```python
from build123d import *

# Parameters (mm, degrees)
SKETCH_1_W                    = 380
SKETCH_1_H                    = 380
EXTRUDE_1_DEPTH               = 14
CHAMFER_1_SIZE                = 2
HOLE_WIZARD_M8_1_D            = 6.8
HOLE_WIZARD_M10_1_D           = 11
HOLE_WIZARD_M10_1_CBORE_D     = 22
HOLE_WIZARD_M10_1_CBORE_DEPTH = 10.5
SKETCH_6_R                    = 8
CUT_EXTRUDE_1_DEPTH           = 15


with BuildPart() as part:
    # 草图1 → 凸台-拉伸1 (new body)
    with BuildSketch(Plane(origin=(0, 0, 0), x_dir=(1, 0, 0), z_dir=(0, 1, 0))):
        Rectangle(SKETCH_1_W, SKETCH_1_H)
    extrude(amount=EXTRUDE_1_DEPTH)

    # 倒角1
    chamfer_1_edges = [part.edges().sort_by_distance(p)[0] for p in [
        (-190, 7, -190),
        (190, 7, -190),
        (190, 7, 190),
        (-190, 7, 190),
    ]]
    chamfer(chamfer_1_edges, length=CHAMFER_1_SIZE)

    # M8 螺纹孔的螺纹孔钻头1 (through all)
    with Locations(Plane(origin=(0, 14, 0), x_dir=(1, 0, 0), z_dir=(0, 1, 0))):
        with Locations((60, 40), (60, 0), (60, -40)):
            hole_wizard_m8_1 = Hole(HOLE_WIZARD_M8_1_D / 2)

    # 镜向1: M8 螺纹孔的螺纹孔钻头1 across plane
    add(hole_wizard_m8_1.mirror(Plane(origin=(0, 0, 0), x_dir=(0, 0, 1), z_dir=(1, 0, 0))), mode=Mode.SUBTRACT)

    # M10 六角头螺栓的柱形沉头孔1 (through all)
    with Locations(Plane(origin=(0, 0, 0), x_dir=(-1, 0, 0), z_dir=(0, -1, 0))):
        with Locations((33.5, 53.5), (-33.5, -13.5), (33.5, -53.5), (-33.5, 53.5), (-33.5, -53.5), (33.5, 13.5)):
            CounterBoreHole(HOLE_WIZARD_M10_1_D / 2, HOLE_WIZARD_M10_1_CBORE_D / 2, HOLE_WIZARD_M10_1_CBORE_DEPTH)

    # 草图6 → 切除-拉伸1 (cut, through all)
    with BuildSketch(Plane(origin=(0, 14, 0), x_dir=(1, 0, 0), z_dir=(0, 1, 0))):
        with Locations((-162, 162)):
            Circle(SKETCH_6_R)
        with Locations((162, 162)):
            Circle(SKETCH_6_R)
        with Locations((-162, -162)):
            Circle(SKETCH_6_R)
        with Locations((162, -162)):
            Circle(SKETCH_6_R)
    extrude(amount=-CUT_EXTRUDE_1_DEPTH, mode=Mode.SUBTRACT)


solid = part.part
```
Read the model definition and answer for the solid it produces. Units are mm, in the model's axes. A direction names the side the tool comes from. Give positions to 0.01 mm unless a question says otherwise; leave off trailing zeros. Write each loop counter-clockwise with the first axis right and the second up, starting at its lowest first coordinate (ties: lowest second). Pieces come first, ordered by that corner, then holes. Notation, with made-up numbers: M 48,-19.5 L 74,-19.5 A21 cw 74,12.5 Z; hole C 65.5,-20.75 d7. An arc over 180 degrees is marked long. Put each result on its own line as item: value. Start each with the question number.
1. The part is cut by section C-C, the plane y = 8. Give the number of separate pieces and of enclosed holes in the cut face, and give its area (3 significant figures).
2. The part is cut by section B-B, the plane x = 162. Give the vertices of the cut face in (y, z), and give its area (3 significant figures).
3. Each of these flat-tipped pins is pushed along its axis until it touches: pin 1 Ø13 at (x, z) = (-162, 162) entering from -Y; pin 2 Ø24 at (x, z) = (32.5, 12.5) entering from -Y; pin 3 Ø20 at (x, z) = (-33.5, -53.5) entering from -Y. Where does it stop, or does it pass through?
4. The part is cut by section D-D, the plane x = -33.5. Give the vertices of the cut face in (y, z).
5. Which of the six approach directions +Z, -Z, +X, -X, +Y, -Y give full straight-line access (tool end or side, diameter ignored) to faces 1 (the cylindrical face through (-38.995, 12.274, -53.742)), 2 (the flat face through (-28, 10.5, -51))?
6. Consider line 1 along Z through (x, y) = (-33.5, 4.5); line 2 along Z through (x, y) = (-60, 9.75); line 3 along X through (y, z) = (13.35, -53.5). Determine where each line is inside the solid, lowest interval first.
7. The part is cut by section A-A, the plane z = 162. Give the vertices of the cut face in (x, y).
Final values:
1. separate pieces: 1
1. enclosed holes: 16
1. area: 141,000 mm²
2. outline: M 0,-190 L 14,-190 L 14,-170 L 0,-170 Z; M 0,-154 L 14,-154 L 14,154 L 0,154 Z; M 0,170 L 14,170 L 14,190 L 0,190 Z
2. area: 4,870 mm²
3. pin 1: passes through
3. pin 2: stops at y = 0
3. pin 3: stops at y = 10.5
4. outline: M 0,-190 L 14,-190 L 14,-59 L 10.5,-59 L 10.5,-64.5 L 0,-64.5 Z; M 0,-42.5 L 10.5,-42.5 L 10.5,-48 L 14,-48 L 14,-19 L 10.5,-19 L 10.5,-24.5 L 0,-24.5 Z; M 0,-2.5 L 10.5,-2.5 L 10.5,-8 L 14,-8 L 14,48 L 10.5,48 L 10.5,42.5 L 0,42.5 Z; M 0,64.5 L 10.5,64.5 L 10.5,59 L 14,59 L 14,190 L 0,190 Z
5. face 1: +Y, -Y
5. face 2: -Y
6. line 1: z = -190 to -64.5, -42.5 to -24.5, -2.5 to 42.5, 64.5 to 190
6. line 2: z = -190 to -43.4, -36.6 to -3.4, 3.4 to 36.6, 43.4 to 190
6. line 3: x = -190 to -39, -28 to 28, 39 to 190
7. outline: M -190,0 L -170,0 L -170,14 L -190,14 Z; M -154,0 L 154,0 L 154,14 L -154,14 Z; M 170,0 L 190,0 L 190,14 L 170,14 Z
